The figure shows three views and two pictorial views of one solid part (mm, origin at its lowest corner). Answer the questions. A direction names the side the tool comes from. Give positions to 0.01 mm unless a question says otherwise; leave off trailing zeros. Write each loop counter-clockwise with the first axis right and the second up, starting at its lowest first coordinate (ties: lowest second). Pieces come first, ordered by that corner, then holes. Notation, with made-up numbers: (76.25, -6) -> (115.25, -6) arc R13 ccw to (115.25, 1) -> close; hole circle Ø4 at (74, -2). An arc over 180 degrees is marked (long way). Answer as CSV lines item,"result". Start each with the question number.
1. The part is cut by section D-D, the plane x = 16.25. Determine the outline of the cut face in (y, z), and give its area (3 significant figures).
2. The part is cut by section B-B, the plane x = 7.25. Determine the outline of the cut face in (y, z).
3. Given pin 1 (11 mm diameter, centred on y = 3, z = 6.5, fed in from +X); pin 2 (8 mm diameter, centred on x = 15, z = 6, fed in from -Y); pin 3 (11 mm diameter, centred on x = 16.5, y = 12.5, fed in from +Z), each flat-ended and moving along its own axis, determine where each tip first touches the part or whether it passes through.
4. Find the intervals of material crossed by line 1 (X direction, y = 2, z = 6.75); line 2 (Y direction, x = 6.75, z = 15), in increasing order.
5. The part is cut by section A-A, the plane z = 1.25. Determine the outline of the cut face in (x, y), and give its area (3 significant figures).
6. The part is cut by section C-C, the plane y = 8. Determine the outline of the cut face in (x, z).
7. A tool of negligible diameter and unlimited length cuts with its end or side. For the marked faces 1, 2, 3 and 4, from which of +Z, -Z, +X, -X, +Y, -Y can it reach the whole face along a straight path? Write none if from no direction.
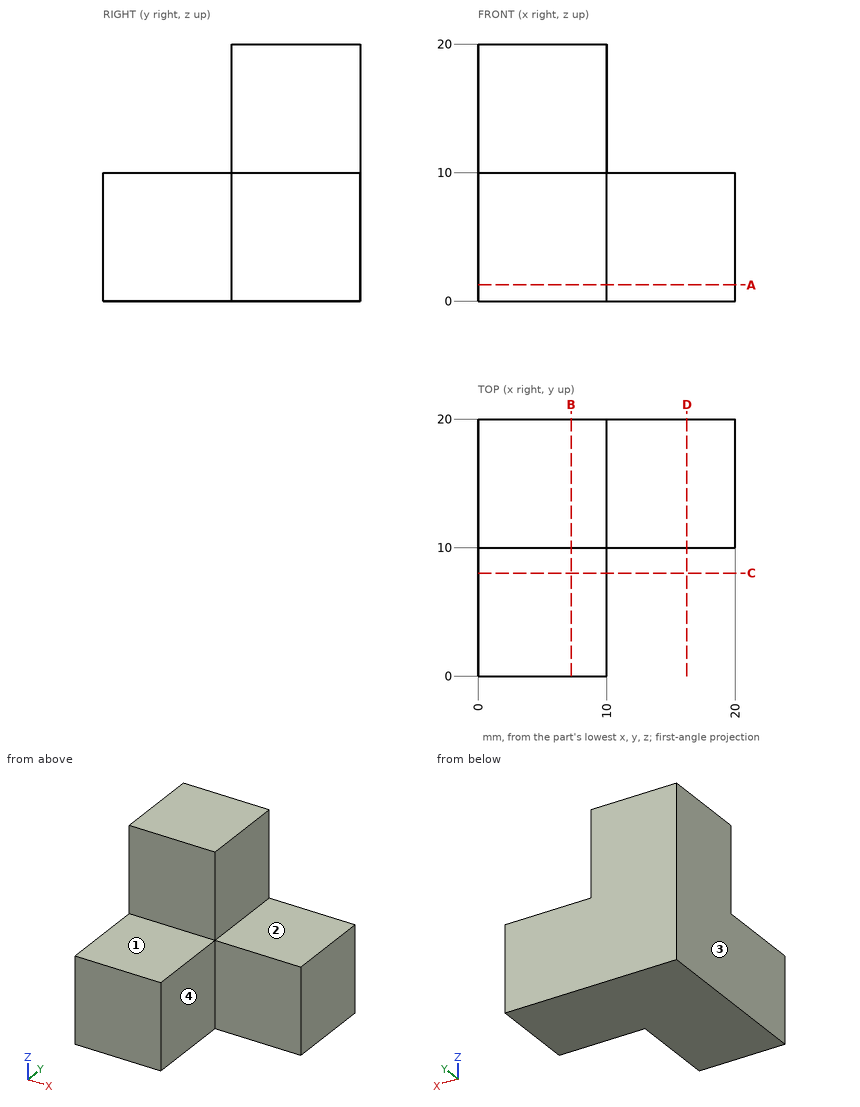
Results found:
1,outline,"(10, 0) -> (20, 0) -> (20, 10) -> (10, 10) -> close"
1,area,"100 mm²"
2,outline,"(0, 0) -> (20, 0) -> (20, 20) -> (10, 20) -> (10, 10) -> (0, 10) -> close"
3,pin 1,"stops at x = 10"
3,pin 2,"stops at y = 10"
3,pin 3,"stops at z = 10"
4,line 1,"x = 0 to 10"
4,line 2,"y = 10 to 20"
5,outline,"(0, 0) -> (10, 0) -> (10, 10) -> (20, 10) -> (20, 20) -> (0, 20) -> close"
5,area,"300 mm²"
6,outline,"(0, 0) -> (10, 0) -> (10, 10) -> (0, 10) -> close"
7,face 1,"+Z, +X, -X, -Y"
7,face 2,"+Z, +X, +Y, -Y"
7,face 3,"+Z, -Z, -X, +Y, -Y"
7,face 4,"+Z, -Z, +X, -Y"
